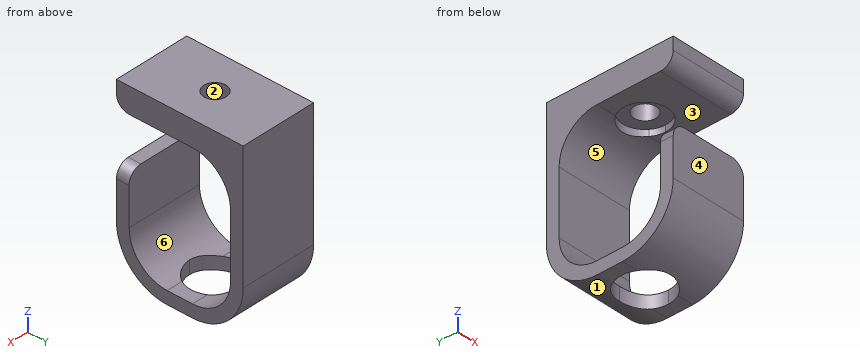
from build123d import *

# Parameters (mm, degrees)
F0_W     = 3.175
F0_H     = 6.35
F1_DEPTH = 9.525
F2_W     = 12.7
F2_H     = 6.35
F2_H_2   = 3.175
F3_DEPTH = 3.7207438789
F4_R     = 6.34999
F5_R     = 3.175
F6_R     = 2.778125
F7_DEPTH = 6.35
F8_R     = 2.778125
F9_DEPTH = 1.5875


# Not quite as in the source:
# - a fillet or chamfer is up to 0.001 mm smaller than in the source, because OpenCascade refuses the exact size
# - a feature names something its author has since deleted; it is built from what else it names


with BuildPart() as f1:
    # F0 (on Right) → F1 (new body, symmetric)
    with BuildSketch(Plane.YZ):
        with BuildLine():
            Line((31.75, 44.45), (3.175, 44.45))
            Line((3.175, 44.45), (3.175, 38.1))
            Line((3.175, 38.1), (19.05, 38.1))
            Line((19.05, 38.1), (28.575, 38.1))
            Line((28.575, 38.1), (28.575, 28.575))
            Line((28.575, 28.575), (28.575, 12.7))
            Line((28.575, 12.7), (28.575, 4.2997395874))
            ThreePointArc((28.575, 4.2997395874), (30.929762203, 8.2098719395), (31.75, 12.7))
            Line((31.75, 12.7), (31.75, 44.45))
        make_face()
        with Locations((1.5875, 41.275)):
            Rectangle(F0_W, F0_H)
        with BuildLine():
            Line((28.575, 38.1), (19.05, 38.1))
            ThreePointArc((19.05, 38.1), (25.7851920908, 35.3101920908), (28.575, 28.575))
            Line((28.575, 28.575), (28.575, 38.1))
        make_face()
        with BuildLine():
            ThreePointArc((27.4502604126, 3.175), (28.0302561211, 3.7197438789), (28.575, 4.2997395874))
            Line((28.575, 4.2997395874), (28.575, 12.7))
            ThreePointArc((28.575, 12.7), (25.7851920908, 5.9648079092), (19.05, 3.175))
            Line((19.05, 3.175), (27.4502604126, 3.175))
        make_face()
        with BuildLine():
            ThreePointArc((19.05, 0), (23.5401280605, 0.820237797), (27.4502604126, 3.175))
            Line((27.4502604126, 3.175), (19.05, 3.175))
            Line((19.05, 3.175), (12.7, 3.175))
            Line((12.7, 3.175), (4.2997395874, 3.175))
            ThreePointArc((4.2997395874, 3.175), (8.2098719395, 0.820237797), (12.7, 0))
            Line((12.7, 0), (19.05, 0))
        make_face()
        with BuildLine():
            ThreePointArc((12.7, 3.175), (5.9648079092, 5.9648079092), (3.175, 12.7))
            Line((3.175, 12.7), (3.175, 4.2997395874))
            ThreePointArc((3.175, 4.2997395874), (3.7197438789, 3.7197438789), (4.2997395874, 3.175))
            Line((4.2997395874, 3.175), (12.7, 3.175))
        make_face()
        with BuildLine():
            Line((3.175, 25.4), (0, 25.4))
            Line((0, 25.4), (0, 12.7))
            ThreePointArc((0, 12.7), (0.820237797, 8.2098719395), (3.175, 4.2997395874))
            Line((3.175, 4.2997395874), (3.175, 12.7))
            Line((3.175, 12.7), (3.175, 25.4))
        make_face()
    extrude(amount=F1_DEPTH, both=True)

    # F2 (on face) → F3 (cut, through all)
    with BuildSketch(Plane(origin=(0, 0, 0), x_dir=(1, 0, 0), z_dir=(0, 0, -1))):
        with Locations((0, -15.875)):
            Rectangle(F2_W, F2_H)
        with Locations((0, -11.1125)):
            Rectangle(F2_W, F2_H_2)
        with Locations((0, -20.6375)):
            Rectangle(F2_W, F2_H_2)
    extrude(amount=-F3_DEPTH, mode=Mode.SUBTRACT)

    # F4 (radius 6.35 in the source; OpenCascade refuses exactly that, so slightly less here)
    f4_edges = [f1.edges().sort_by_distance(p)[0] for p in [
        (-6.35, 22.225, 2.061511),
        (-6.35, 9.525, 2.061511),
        (6.35, 9.525, 2.061511),
        (6.35, 22.225, 2.061511),
    ]]
    fillet(f4_edges, radius=F4_R)

    # F5
    f5_edges = [f1.edges().sort_by_distance(p)[0] for p in [
        (0, 0, 38.1),
        (9.525, 1.5875, 25.4),
        (-9.525, 1.5875, 25.4),
    ]]
    fillet(f5_edges, radius=F5_R)

    # F6 (on face) → F7 (cut, through all)
    with BuildSketch(Plane.XY.offset(44.45)):
        with Locations((0, 15.875)):
            Circle(F6_R)
    extrude(amount=-F7_DEPTH, mode=Mode.SUBTRACT)

    # F8 (on face) → F9 (cut, symmetric)
    with BuildSketch(Plane(origin=(0, 0, 38.1), x_dir=(1, 0, 0), z_dir=(0, 0, -1))):
        with BuildLine():
            ThreePointArc((4.5597466007, -19.05), (5.3012737202, -17.5388542623), (5.55625, -15.875))
            ThreePointArc((5.55625, -15.875), (-1.6638542623, -10.5737262798), (-4.5597466007, -19.05))
            Line((-4.5597466007, -19.05), (4.5597466007, -19.05))
        make_face()
        with Locations((0, -15.875)):
            Circle(F8_R, mode=Mode.SUBTRACT)
        with BuildLine():
            Line((4.5597466007, -19.05), (-4.5597466007, -19.05))
            ThreePointArc((-4.5597466007, -19.05), (0, -21.43125), (4.5597466007, -19.05))
        make_face()
    extrude(amount=F9_DEPTH, both=True, mode=Mode.SUBTRACT)


solid = f1.part
Check sheet for the modelled part. Datum: model origin and axes. Units: mm. Face numbers are marked on the shaded views. A direction names the side the tool comes from. Round coordinates to 2 decimals unless told otherwise and drop trailing zeros. Loops run counter-clockwise (first coordinate to the right, second up) from the corner with the lowest first, then second, coordinate; pieces in that order, holes last.
1. Sectioned sample at A-A on z = 42. Record the boundary of the cut face in (x, y) (3 decimals).
2. Gauge pin test, flat ends, axial feed: pin 1 Ø6 at (y, z) = (14.5, 35) entering from -X; pin 2 Ø2 at (x, y) = (-4.5, 5) entering from -Z; pin 3 Ø10 at (x, y) = (0.5, 27) entering from -Z; pin 4 Ø9 at (x, y) = (0, 15.875) entering from -Z. Record the tip position at first contact, or that the pin passes through.
3. Scan lines: probe 1 along Z at (x, y) = (-8.25, 18) (3 decimals); probe 2 along Y at (x, z) = (0, 41.7); probe 3 along Z at (x, y) = (1.25, 20). Record each from-to range of solid material in increasing order.
4. Set-up check for the marked faces 4, 5 and 6: record each of +Z, -Z, +X, -X, +Y, -Y from which the full face is reachable in a straight line by a thin tool's end or side.
5. Mould release check, pull along Z, two halves, no side actions. Record for the marked faces 1, 2 and 3: released by +Z, released by -Z, zero draft, split by the parting line, or undercut.
6. Sectioned sample at C-C on x = -0.5. Give the number of separate pieces and of enclosed holes in the cut face, and give its area (3 significant figures).
7. Sectioned sample at B-B on z = 5.5. Record the boundary of the cut face in (x, y) (3 decimals), and give its area (3 significant figures).
Recorded:
1. outline: (-9.525, 0) - (9.525, 0) - (9.525, 31.75) - (-9.525, 31.75) - close; hole circle Ø5.556 at (0, 15.875)
2. pin 1: passes through
2. pin 2: stops at z = 1.91
2. pin 3: stops at z = 0.37
2. pin 4: stops at z = 39.69
3. probe 1: z = 0 to 3.175, 38.1 to 44.45
3. probe 2: y = 0 to 13.1, 18.65 to 31.75
3. probe 3: z = 39.69 to 44.45
4. face 4: +Z, -Z, +X, -X, -Y
4. face 5: +X, -X, -Y
4. face 6: +X, -X
5. face 1: released by -Z
5. face 2: zero draft
5. face 3: undercut
6. separate pieces: 3
6. enclosed holes: 0
6. area: 387 mm2
7. outline: (-9.525, 2.238) - (9.525, 2.238) - (9.525, 6.464) - (-9.525, 6.464) - close; (-9.525, 25.286) - (9.525, 25.286) - (9.525, 29.512) - (-9.525, 29.512) - close
7. area: 161 mm2
